```python
from build123d import *

# Parameters (mm, degrees)
F1_DEPTH = 127
F2_R     = 5.08


with BuildPart() as f1:
    # F0 (on Front) → F1 (new body)
    with BuildSketch(Plane.XZ):
        Polygon((-30.983802, 42.413801), (-57.244465, 44.491984), (-57.244465, 9.162893), (-28.338844, 9.162893), align=None)
    extrude(amount=F1_DEPTH)

    # F2
    f2_edges = [f1.edges().sort_by_distance(p)[0] for p in [
        (-30.983802, -63.5, 42.413801),
        (-57.244465, -63.5, 44.491984),
        (-44.114133, -127, 43.452892),
        (-29.661323, -127, 25.788347),
        (-42.791654, -127, 9.162893),
        (-57.244465, -127, 26.827438),
        (-28.338844, -63.5, 9.162893),
        (-57.244465, -63.5, 9.162893),
        (-29.661323, 0, 25.788347),
        (-44.114133, 0, 43.452892),
        (-57.244465, 0, 26.827438),
        (-42.791654, 0, 9.162893),
    ]]
    fillet(f2_edges, radius=F2_R)


solid = f1.part
```
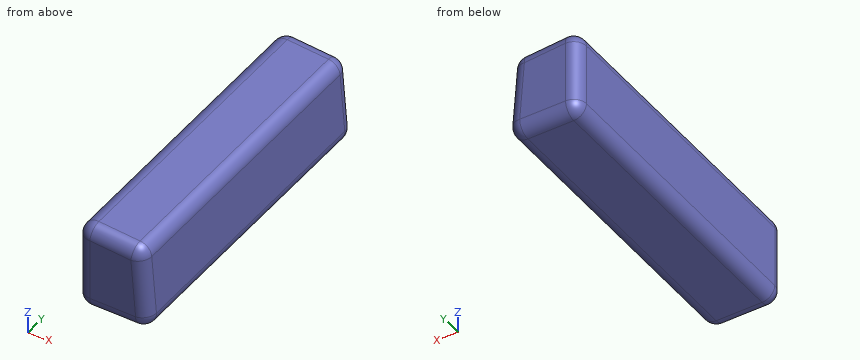
Geometry: final body of the model. Coordinates: model frame, mm. Coordinates: 2 decimals unless noted, no trailing zeros. Order: outer loops, then holes, each group sorted by start corner. A loop starts at its lowest first (then second) coordinate and runs counter-clockwise, first axis right, second up. Notation, with made-up numbers: M 41,18 L 82,18 A10 ccw 82,26 Z; hole C 6.25,-21.5 d9. An arc over 180 degrees is marked long. Answer in a Markdown table with one row per item. Add a question column.
Q1. Contact query for flat-ended pins moving along their axis: P1, Ø3, axis at y = -65.5, z = 37.5, coming from the +X side; P2, Ø12, axis at y = -78, z = 30, coming from the +X side. Output: stop coordinate, or through.
Q2. Section query A-A on y = -63.5. Return the cut outline in (x, z).
Q3. Section query B-B on x = -53.5. Return the cut outline in (y, z).
Q4. Line query: L1, parallel to Y at x = -52.5, z = 22; L2, parallel to Z at x = -52.25, y = -56.5; L3, parallel to X at y = -49.5, z = 15. Output: solid intervals per line, ascending.
Completed:
| question | item | result |
|---|---|---|
| 1 | P1 | stops at x = -30.47 |
| 1 | P2 | stops at x = -29.52 |
| 2 | outline | M -57.24,14.24 A5.08 ccw -52.16,9.16 L -33.84,9.16 A5.08 ccw -28.77,14.65 L -30.64,38.09 A5.08 ccw -35.3,42.76 L -51.76,44.06 A5.08 ccw -57.24,38.99 Z |
| 3 | outline | M -126.82,14.24 A4.9 ccw -121.92,9.34 L -5.08,9.34 A4.9 ccw -0.18,14.24 L -0.18,38.99 A4.9 ccw -5.08,43.9 L -121.92,43.9 A4.9 ccw -126.82,38.99 Z |
| 4 | L1 | y = -126.99 to -0.01 |
| 4 | L2 | z = 9.16 to 44.07 |
| 4 | L3 | x = -57.24 to -28.8 |
